Read the model definition and answer for the solid it produces. Units are mm, in the model's axes. Face numbers are marked on the shaded views. A direction names the side the tool comes from. Give positions to 0.01 mm unless a question says otherwise; leave off trailing zeros. Write each loop counter-clockwise with the first axis right and the second up, starting at its lowest first coordinate (ties: lowest second). Pieces come first, ordered by that corner, then holes. Notation, with made-up numbers: (7, 33.25) - (58, 33.25) arc R11 ccw to (58, 43.25) - close; hole circle Ø4 at (10.25, 55.5). An arc over 180 degrees is marked (long way). Answer as CSV lines item,"result".
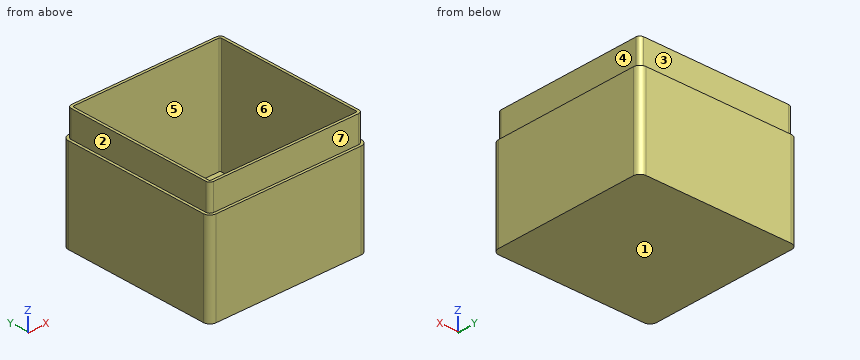
```python
from build123d import *

# Parameters (mm, degrees)
SKETCH1_W           = 120
SKETCH1_H           = 120
BOSS_EXTRUDE1_DEPTH = 90
FILLET1_R           = 5
SHELL1_T            = -4
CUT_EXTRUDE2_DEPTH  = 20


with BuildPart() as part:
    # Sketch1 → Boss-Extrude1 (new body)
    with BuildSketch(Plane.XY):
        with Locations((60, 60)):
            Rectangle(SKETCH1_W, SKETCH1_H)
    extrude(amount=BOSS_EXTRUDE1_DEPTH)

    # Fillet1
    fillet1_edges = [part.edges().sort_by_distance(p)[0] for p in [
        (0, 120, 45),
        (120, 120, 45),
        (120, 0, 45),
        (0, 0, 45),
    ]]
    fillet(fillet1_edges, radius=FILLET1_R)

    # Shell1
    shell1_openings = [part.faces().sort_by_distance(p)[0] for p in [
        (60, 60, 90),
    ]]
    offset(amount=SHELL1_T, openings=shell1_openings, kind=Kind.INTERSECTION)

    # Sketch8 → Cut-Extrude2 (cut)
    with BuildSketch(Plane.XY.offset(90)):
        with BuildLine():
            Line((120, 5), (120, 115))
            ThreePointArc((120, 115), (118.535533906, 118.535533906), (115, 120))
            Line((115, 120), (5, 120))
            ThreePointArc((5, 120), (1.464466094, 118.535533906), (0, 115))
            Line((0, 115), (0, 5))
            ThreePointArc((0, 5), (1.464466094, 1.464466094), (5, 0))
            Line((5, 0), (115, 0))
            ThreePointArc((115, 0), (118.535533906, 1.464466094), (120, 5))
        make_face()
        with BuildLine():
            Line((118, 5), (118, 115))
            ThreePointArc((118, 115), (117.121320344, 117.121320344), (115, 118))
            Line((115, 118), (5, 118))
            ThreePointArc((5, 118), (2.878679656, 117.121320344), (2, 115))
            Line((2, 115), (2, 5))
            ThreePointArc((2, 5), (2.878679656, 2.878679656), (5, 2))
            Line((5, 2), (115, 2))
            ThreePointArc((115, 2), (117.121320344, 2.878679656), (118, 5))
        make_face(mode=Mode.SUBTRACT)
    extrude(amount=-CUT_EXTRUDE2_DEPTH, mode=Mode.SUBTRACT)


solid = part.part
```
(1) The mould has two halves that part along Y. Classify the marked faces 4, 5, 6 and 7: +Y half, -Y half, draft (parallel to the pull), parting line (faces both ways), or undercut.
Worked out:
face 4,"draft"
face 5,"undercut"
face 6,"undercut"
face 7,"-Y half"
(2) A cutting plane is placed at A-A (z = 72.5). Write down the section's boundary in (x, y).
Worked out:
outline,"(2, 5) arc R3 ccw to (5, 2) - (115, 2) arc R3 ccw to (118, 5) - (118, 115) arc R3 ccw to (115, 118) - (5, 118) arc R3 ccw to (2, 115) - close; hole (4, 5) arc R1 ccw to (5, 4) - (115, 4) arc R1 ccw to (116, 5) - (116, 115) arc R1 ccw to (115, 116) - (5, 116) arc R1 ccw to (4, 115) - close"
(3) Find the intervals of material crossed by L1, parallel to Y at x = 27.5, z = 33.5; L2, parallel to Y at x = 73.5, z = 84.5, in increasing order.
Worked out:
L1,"y = 0 to 4, 116 to 120"
L2,"y = 2 to 4, 116 to 118"
(4) For the marked faces 1, 2 and 3, determine the directions among +Z, -Z, +X, -X, +Y, -Y from which every point of the face is accessible in a straight line to the end or side of a thin tool.
Worked out:
face 1,"-Z, +X, -X, +Y, -Y"
face 2,"+Z, -X, +Y, -Y"
face 3,"+Z, +X, -X, +Y"
(5) A cutting plane is placed at B-B (x = 29). Write down the section's boundary in (y, z).
Worked out:
outline,"(0, 0) - (120, 0) - (120, 70) - (118, 70) - (118, 90) - (116, 90) - (116, 4) - (4, 4) - (4, 90) - (2, 90) - (2, 70) - (0, 70) - close"
(6) Each of these flat-tipped pins is pushed along its axis until it touches: P1, Ø6, axis at x = 58, z = 83, coming from the +Y side; P2, Ø16, axis at y = 74.5, z = 84.5, coming from the -X side; P3, Ø1, axis at x = 52.5, y = 82, coming from the +Z side. Where does it stop, or does it pass through?
Worked out:
P1,"stops at y = 118"
P2,"stops at x = 2"
P3,"stops at z = 4"
(7) A cutting plane is placed at D-D (z = 52.5). Write down the section's boundary in (x, y).
Worked out:
outline,"(0, 5) arc R5 ccw to (5, 0) - (115, 0) arc R5 ccw to (120, 5) - (120, 115) arc R5 ccw to (115, 120) - (5, 120) arc R5 ccw to (0, 115) - close; hole (4, 5) arc R1 ccw to (5, 4) - (115, 4) arc R1 ccw to (116, 5) - (116, 115) arc R1 ccw to (115, 116) - (5, 116) arc R1 ccw to (4, 115) - close"
